Geometry: see drawing. Coordinates: mm, zero at the bounding-box minimum. A direction names the side the tool comes from. Give positions to 0.01 mm unless a question says otherwise; leave off trailing zeros. Write each loop counter-clockwise with the first axis right and the second up, starting at its lowest first coordinate (ties: lowest second). Pieces come first, ordered by that corner, then holes. Notation, with made-up numbers: M -12.75,-29 L 42.25,-29 A18 ccw 42.25,-10 Z; hole C 52.25,-1 d9. An arc over 180 degrees is marked long. Use CSV: the item, a comma, the result in double quotes. Start each with the question number.
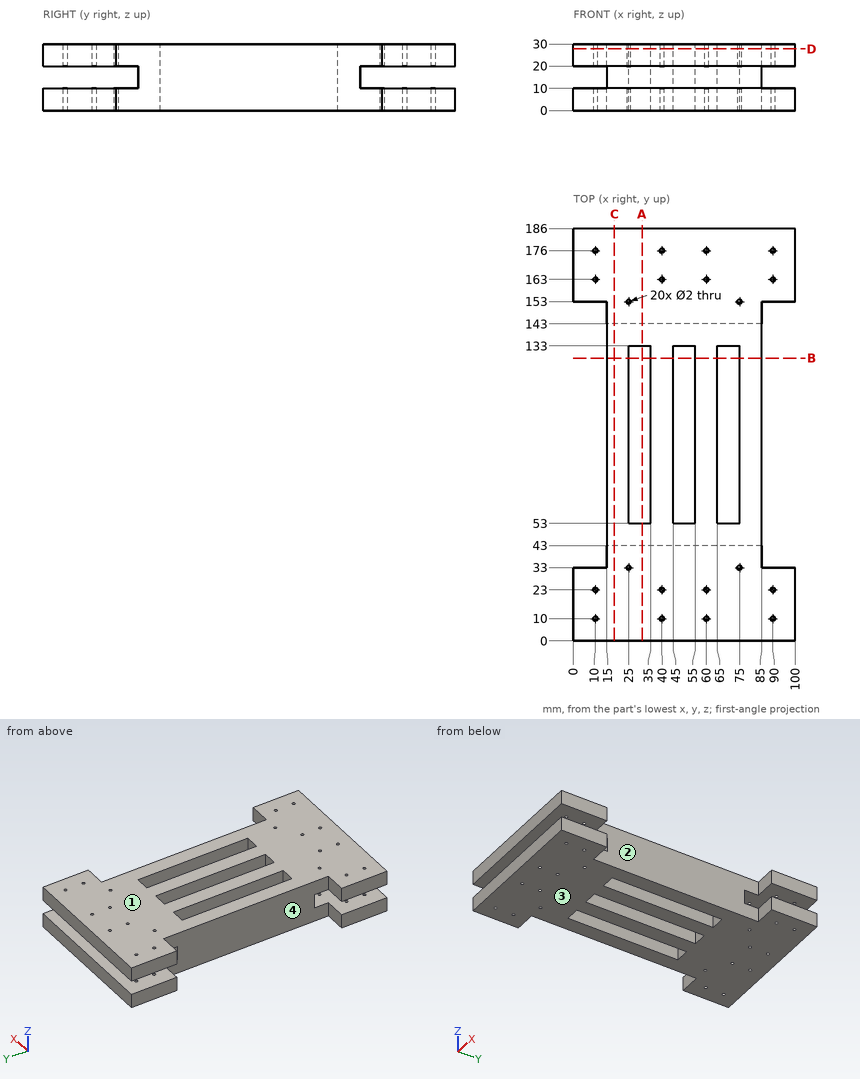
1. Pull-direction query (Y, two-part tool) for the marked faces 1 and 2; classes: released by +Y, released by -Y, zero draft, split by the parting line, or undercut.
2. Section B-B on y = 127.5. Return loops of the section in (x, z).
3. First-contact query: pin 1 (8 mm diameter, centred on y = 73.5, z = 22.5, fed in from +X); pin 2 (3 mm diameter, centred on x = 70.5, z = 11, fed in from -Y); pin 3 (1.6 mm diameter, centred on x = 90, y = 23, fed in from -Z); pin 4 (1 mm diameter, centred on y = 61.5, z = 17, fed in from -X). Flat tips, straight axial feed; report the tip coordinate or a pass-through.
4. Section C-C on x = 18.5. Return loops of the section in (y, z), then the cut area to 3 significant figures.
5. Line query: probe 1 along X at (y, z) = (124, 15.5); probe 2 along Y at (x, z) = (40, 2.5); probe 3 along Y at (x, z) = (90, 4.75). Output: solid intervals per line, ascending.
6. Access query for the marked faces 3 and 4. Directions: +Z, -Z, +X, -X, +Y, -Y. A direction counts if a zero-diameter tool reaches every point of the face in a straight line with its end or side. Return the directions, or none.
7. Section D-D on z = 27.75. Give the number of separate pieces and of enclosed holes in the cut face, then the cut area to 3 significant figures.
8. Section A-A on x = 31. Return loops of the section in (y, z).
Resolved:
1,face 1,"zero draft"
1,face 2,"undercut"
2,outline,"M 15,0 L 25,0 L 25,30 L 15,30 Z; M 35,0 L 45,0 L 45,30 L 35,30 Z; M 55,0 L 65,0 L 65,30 L 55,30 Z; M 75,0 L 85,0 L 85,30 L 75,30 Z"
3,pin 1,"stops at x = 85"
3,pin 2,"stops at y = 0"
3,pin 3,"passes through"
3,pin 4,"stops at x = 15"
4,outline,"M 0,0 L 186,0 L 186,10 L 143,10 L 143,20 L 186,20 L 186,30 L 0,30 L 0,20 L 43,20 L 43,10 L 0,10 Z"
4,area,"4,720 mm2"
5,probe 1,"x = 15 to 25, 35 to 45, 55 to 65, 75 to 85"
5,probe 2,"y = 0 to 9, 11 to 22, 24 to 162, 164 to 175, 177 to 186"
5,probe 3,"y = 0 to 9, 11 to 22, 24 to 33, 153 to 162, 164 to 175, 177 to 186"
6,face 3,"-Z, +X, -X, +Y, -Y"
6,face 4,"+Z, -Z, -X"
7,separate pieces,"1"
7,enclosed holes,"23"
7,area,"12,500 mm2"
8,outline,"M 0,0 L 53,0 L 53,30 L 0,30 L 0,20 L 43,20 L 43,10 L 0,10 Z; M 133,0 L 186,0 L 186,10 L 143,10 L 143,20 L 186,20 L 186,30 L 133,30 Z"
